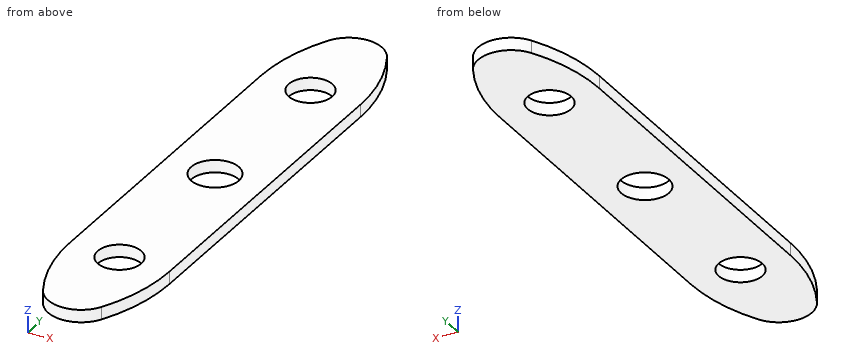
```python
from build123d import *

# Parameters (mm, degrees)
SKETCH1_R          = 9.128125
SKETCH1_R_2        = 8.334375
BASE_EXTRUDE_DEPTH = 4.7752


with BuildPart() as part:
    # Sketch1 → Base-Extrude (new body)
    with BuildSketch(Plane.XY):
        with BuildLine():
            Line((19.05, 63.5), (19.05, -63.5))
            ThreePointArc((19.05, -63.5), (17.059251197, -79.671062799), (11.205882353, -94.876470588))
            ThreePointArc((11.205882353, -94.876470588), (0, -101.6), (-11.205882353, -94.876470588))
            ThreePointArc((-11.205882353, -94.876470588), (-17.059251197, -79.671062799), (-19.05, -63.5))
            Line((-19.05, -63.5), (-19.05, 63.5))
            ThreePointArc((-19.05, 63.5), (-17.059251197, 79.671062799), (-11.205882353, 94.876470588))
            ThreePointArc((-11.205882353, 94.876470588), (0, 101.6), (11.205882353, 94.876470588))
            ThreePointArc((11.205882353, 94.876470588), (17.059251197, 79.671062799), (19.05, 63.5))
        make_face()
        Circle(SKETCH1_R, mode=Mode.SUBTRACT)
        with Locations((0, -63.5)):
            Circle(SKETCH1_R_2, mode=Mode.SUBTRACT)
        with Locations((0, 63.5)):
            Circle(SKETCH1_R_2, mode=Mode.SUBTRACT)
    extrude(amount=BASE_EXTRUDE_DEPTH)


solid = part.part
```
Check sheet for the modelled part. Datum: model origin and axes. Units: mm. Round coordinates to 2 decimals unless told otherwise and drop trailing zeros. Order: outer loops, then holes, each group sorted by start corner. A loop starts at its lowest first (then second) coordinate and runs counter-clockwise, first axis right, second up. Notation, with made-up numbers: (-5, -30) -> (25, -30) arc R23 cw to (25, -4) -> close; hole circle Ø4 at (-5, 5.5). An arc over 180 degrees is marked (long way). One line per item, written item: value. Start each with the question number.
Q1. Thickness scan on line 1 (Y direction, x = 0, z = 2.35); line 2 (Y direction, x = 2, z = 1.9); line 3 (X direction, y = -2.5, z = 4.4). Record the ranges inside material, lowest first.
Q2. Cross-section at D-D (y = 0). Record the boundary of the cut face in (x, z), and give its area (3 significant figures).
Q3. Cross-section at B-B (y = 57). Record the boundary of the cut face in (x, z), and give its area (3 significant figures).
Q4. Cross-section at A-A (z = 3.35). Record the boundary of the cut face in (x, y) (3 decimals).
Q5. Gauge pin test, flat end, axial feed: pin 1 Ø2 at (x, z) = (-9.5, 4) entering from -Y. Record the tip position at first contact, or that the pin passes through.
Q6. Cross-section at C-C (x = 6). Record the boundary of the cut face in (y, z), and give its area (3 significant figures).
Completed:
1. line 1: y = -101.6 to -71.83, -55.17 to -9.13, 9.13 to 55.17, 71.83 to 101.6
1. line 2: y = -101.44 to -71.59, -55.41 to -8.91, 8.91 to 55.41, 71.59 to 101.44
1. line 3: x = -19.05 to -8.78, 8.78 to 19.05
2. outline: (-19.05, 0) -> (-9.13, 0) -> (-9.13, 4.78) -> (-19.05, 4.78) -> close; (9.13, 0) -> (19.05, 0) -> (19.05, 4.78) -> (9.13, 4.78) -> close
2. area: 94.8 mm²
3. outline: (-19.05, 0) -> (-5.22, 0) -> (-5.22, 4.78) -> (-19.05, 4.78) -> close; (5.22, 0) -> (19.05, 0) -> (19.05, 4.78) -> (5.22, 4.78) -> close
3. area: 132 mm²
4. outline: (-19.05, -63.5) arc R66.675 ccw to (-11.206, -94.876) arc R12.7 ccw to (11.206, -94.876) arc R66.675 ccw to (19.05, -63.5) -> (19.05, 63.5) arc R66.675 ccw to (11.206, 94.876) arc R12.7 ccw to (-11.206, 94.876) arc R66.675 ccw to (-19.05, 63.5) -> close; hole circle Ø18.256 at (0, 0); hole circle Ø16.669 at (0, -63.5); hole circle Ø16.669 at (0, 63.5)
5. pin 1: stops at y = -98.34
6. outline: (-100.09, 0) -> (-69.28, 0) -> (-69.28, 4.78) -> (-100.09, 4.78) -> close; (-57.72, 0) -> (-6.88, 0) -> (-6.88, 4.78) -> (-57.72, 4.78) -> close; (6.88, 0) -> (57.72, 0) -> (57.72, 4.78) -> (6.88, 4.78) -> close; (69.28, 0) -> (100.09, 0) -> (100.09, 4.78) -> (69.28, 4.78) -> close
6. area: 780 mm²
